Solid Edge part; units mm, degrees
sketch "Sketch1" plane through (0, 0, 0) normal (0, 0, 1) x (1, 0, 0)
  line L0 (23.4, 6) -> (20.4, 6)
  line L1 (20.4, 6) -> (20.4, 10.6667)
  line L2 (20.4, 10.6667) -> (23.4, 10.6667)
  line L3 (23.4, 10.6667) -> (23.4, 6)
revolve "RevolvedProtrusion1" add sketch "Sketch1" angle 360 about axis through (23.4, 10.6667, 0) along (0, -1, 0)
cosmetic_thread "Thread1"
sketch "Sketch2" plane through (23.4, 10.6667, 0) normal (0, 1, 0) x (-1, 0, 0)
  line L0 (-0.6, 11.985) -> (-0.6, -11.985)
  arc A0 (-0.6, -11.985) -> (0.6, -11.985) centre (0, 0) ccw
  line L1 (0.6, -11.985) -> (0.6, 11.985)
  arc A1 (0.6, 11.985) -> (-0.6, 11.985) centre (0, 0) ccw
extrude "Cutout1" cut sketch "Sketch2" against normal blind 0.6
properties part number "UCP201 GB/T7810-1995_PART6"
Read the model definition and answer for the solid it produces. Units are mm, in the model's axes. A direction names the side the tool comes from. Round coordinates to 2 decimals unless told otherwise and drop trailing zeros. Write each loop counter-clockwise with the first axis right and the second up, starting at its lowest first coordinate (ties: lowest second). Pieces come first, ordered by that corner, then holes.
1. The part is cut by section C-C, the plane z = 0. Determine the outline of the cut face in (x, y), then the cut area to 3 significant figures.
2. The part is cut by section B-B, the plane x = 23.4. Determine the outline of the cut face in (y, z), then the cut area to 3 significant figures.
3. Which of the six approach directions +Z, -Z, +X, -X, +Y, -Y give full straight-line access (tool end or side, diameter ignored) to faces 1 (the face through (22.016, 8.366, -2.662)), 2 (the face through (23, 10.067, 0))?
4. The part is cut by section A-A, the plane z = -2.4. Determine the outline of the cut face in (x, y).
5. Given pin 1 Ø0.7 at (y, z) = (10.5, -1.5) entering from +X, flat-ended and moving along its own axis, determine where the tip first touches the part or whether it passes through.
6. The part is cut by section D-D, the plane y = 8.25. Determine the outline of the cut face in (x, z), then the cut area to 3 significant figures.
7. Straight lines are drawn through the part: L1, parallel to X at y = 10.3, z = -1.1; L2, parallel to Y at x = 23.35, z = -1.9; L3, parallel to X at y = 9, z = 0.2. For each, find the intervals that lie inside material, in ascending order.
Values:
1. outline: (20.4, 6) - (26.4, 6) - (26.4, 10.67) - (24, 10.67) - (24, 10.07) - (22.8, 10.07) - (22.8, 10.67) - (20.4, 10.67) - close
1. area: 27.3 mm2
2. outline: (6, -3) - (10.07, -3) - (10.07, 3) - (6, 3) - close
2. area: 24.4 mm2
3. face 1: +Y, -Y
3. face 2: +Z, -Z, +Y
4. outline: (21.6, 6) - (25.2, 6) - (25.2, 10.67) - (24, 10.67) - (24, 10.07) - (22.8, 10.07) - (22.8, 10.67) - (21.6, 10.67) - close
5. pin 1: stops at x = 26.17
6. outline: circle Ø6 at (23.4, 0)
6. area: 28.3 mm2
7. L1: x = 20.61 to 22.8, 24 to 26.19
7. L2: y = 6 to 10.07
7. L3: x = 20.41 to 26.39
